```python
from build123d import *

# Parameters (mm, degrees)
F1_DEPTH = 2


with BuildPart() as f1:
    # F0 (on Top) → F1 (new body)
    with BuildSketch(Plane.XY):
        with BuildLine():
            ThreePointArc((49.94281, 0.754074), (48.258039, 3.792781), (45, 5))
            Line((45, 5), (-45, 5))
            ThreePointArc((-45, 5), (-48.258039, 3.792781), (-49.94281, 0.754074))
            ThreePointArc((-49.94281, 0.754074), (-49.985682, 0.37812), (-50, 0))
            Line((-50, 0), (-50, -5))
            Line((-50, -5), (-46.019139, -5))
            Line((-46.019139, -5), (-46.019139, -3.395926))
            ThreePointArc((-46.019139, -3.395926), (-41.869139, 0.754074), (-37.719139, -3.395926))
            Line((-37.719139, -3.395926), (-37.719139, -5))
            Line((-37.719139, -5), (-34.719139, -5))
            ThreePointArc((-34.719139, -5), (-33.304926, -4.414214), (-32.719139, -3))
            Line((-32.719139, -3), (-32.719139, -2))
            ThreePointArc((-32.719139, -2), (-32.133353, -0.585786), (-30.719139, 0))
            Line((-30.719139, 0), (32.700289, 0))
            ThreePointArc((32.700289, 0), (34.114502, -0.585786), (34.700289, -2))
            Line((34.700289, -2), (34.700289, -3))
            ThreePointArc((34.700289, -3), (35.286075, -4.414214), (36.700289, -5))
            Line((36.700289, -5), (39.700289, -5))
            Line((39.700289, -5), (39.700289, -2.395926))
            ThreePointArc((39.700289, -2.395926), (42.850289, 0.754074), (46.000289, -2.395926))
            Line((46.000289, -2.395926), (46.000289, -5))
            Line((46.000289, -5), (50, -5))
            Line((50, -5), (50, 0))
            ThreePointArc((50, 0), (49.985682, 0.37812), (49.94281, 0.754074))
        make_face()
    extrude(amount=F1_DEPTH)


solid = f1.part
```
Model file for the job. Use its own axes, mm. A direction names the side the tool comes from. Round coordinates to 2 decimals unless told otherwise and drop trailing zeros. Write each loop counter-clockwise with the first axis right and the second up, starting at its lowest first coordinate (ties: lowest second). Pieces come first, ordered by that corner, then holes. Notation, with made-up numbers: (-38, -8) -> (-34, -8) arc R9 ccw to (-34, 2) -> close; hole circle Ø6 at (-8.5, 72.25). An arc over 180 degrees is marked (long way). Answer as CSV lines item,"result".
1. Mould opens along X. For faces 3 (the face through (-46.019, -4, 1)), 4 (the face through (48, 4, 1)), 5 (the face through (-1, 2, 2)), 6 (the face through (-48, 4, 1)) say: +X half, -X half, draft (parallel to the pull), parting line (faces both ways), or undercut.
Resolved:
face 3,"undercut"
face 4,"+X half"
face 5,"draft"
face 6,"-X half"
2. Slice it at A-A, the plane z = 1.3. List the corners of the cut face in (x, y).
Resolved:
outline,"(-50, -5) -> (-46.02, -5) -> (-46.02, -3.4) arc R4.15 cw to (-37.72, -3.4) -> (-37.72, -5) -> (-34.72, -5) arc R2 ccw to (-32.72, -3) -> (-32.72, -2) arc R2 cw to (-30.72, 0) -> (32.7, 0) arc R2 cw to (34.7, -2) -> (34.7, -3) arc R2 ccw to (36.7, -5) -> (39.7, -5) -> (39.7, -2.4) arc R3.15 cw to (46, -2.4) -> (46, -5) -> (50, -5) -> (50, 0) arc R5 ccw to (49.94, 0.75) arc R5 ccw to (45, 5) -> (-45, 5) arc R5 ccw to (-49.94, 0.75) arc R5 ccw to (-50, 0) -> close"
3. Tool access for faces 1 (the face through (1, 0, 1)), 2 (the face through (48, -5, 1)): list every direction of +Z, -Z, +X, -X, +Y, -Y with a clear straight run to the whole face (end or side of a thin tool).
Resolved:
face 1,"+Z, -Z, -Y"
face 2,"+Z, -Z, +X, -X, -Y"
4. Slice it at B-B, the plane x = -22.5. List the corners of the cut face in (y, z).
Resolved:
outline,"(0, 0) -> (5, 0) -> (5, 2) -> (0, 2) -> close"
5. Drill centre lines: line 1 (X direction, y = -2.25, z = 1.95); line 2 (X direction, y = 0.25, z = 0.1); line 3 (Y direction, x = -10, z = 0.45). Where is each one in solid material? Low to high.
Resolved:
line 1,"-50 to -45.86, -37.88 to -32.72, 34.7 to 39.7, 46 to 50"
line 2,"-49.99 to -43.85, -39.89 to 41.14, 44.56 to 49.99"
line 3,"0 to 5"
6. Pin check, flat tip, straight feed: pin 1 Ø1 at (y, z) = (1.5, 1) entering from +X. Stop position of the tip, or through.
Resolved:
pin 1,"x = 49.9"
